Here's how the part is built. I have some questions about the finished solid (model axes, mm). Coordinates: 2 decimals unless noted, no trailing zeros. Write each loop counter-clockwise with the first axis right and the second up, starting at its lowest first coordinate (ties: lowest second). Pieces come first, ordered by that corner, then holes. Notation, with made-up numbers: (-24, 89.5) -> (10, 89.5) arc R21 cw to (10, 120.5) -> close; hole circle Ø7 at (62.5, -21). An arc over 180 degrees is marked (long way). Use a Markdown table: item, result. Add a question column.
Item 1: Imagine slicing it at A-A, the plane x = 5.75. Write out the boundary of the cut face in (y, z).
Item 2: Will this pin go through, and if not, where does the flat tip stop? pin 1 Ø9 at (x, y) = (11.5, -1519.5) entering from +Z.
Item 3: Imagine slicing it at B-B, the plane y = -153. Write out the boundary of the cut face in (x, z).
Item 4: If I drill on line 1 along Y through (x, z) = (9, 227); line 2 along Z through (x, y) = (15.5, -1504), over which ranges is the centre line in solid material (lowest first)? Write a range as from..to.
```python
from build123d import *

# Parameters (mm, degrees)
F0_W     = 17.78
F0_H     = 241.3
F1_DEPTH = 1778
F2_W     = 177.8
F2_H     = 25.4
F3_DEPTH = 17.781


with BuildPart() as f1:
    # F0 (on Front) → F1 (new body)
    with BuildSketch(Plane.XZ):
        with Locations((8.89, 120.65)):
            Rectangle(F0_W, F0_H)
    extrude(amount=F1_DEPTH)

    # F2 (on face) → F3 (cut, through all)
    with BuildSketch(Plane.YZ.offset(17.78)):
        with Locations((-203.2, 228.6)):
            Rectangle(F2_W, F2_H)
        with Locations((-1555.75, 228.6)):
            Rectangle(F2_W, F2_H)
    extrude(amount=-F3_DEPTH, mode=Mode.SUBTRACT)


solid = f1.part
```
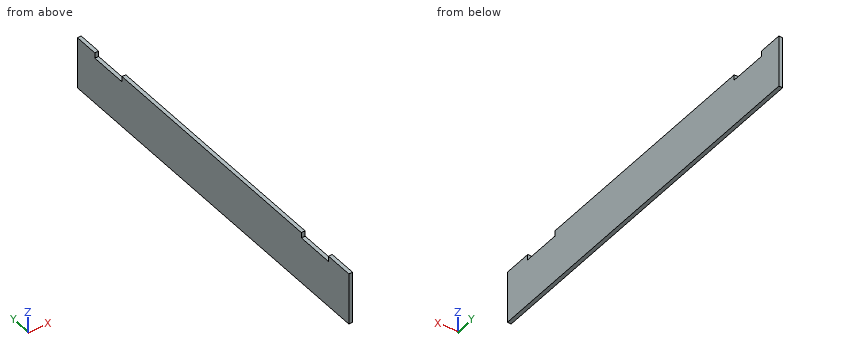
Ans:
| question | item | result |
|---|---|---|
| 1 | outline | (-1778, 0) -> (0, 0) -> (0, 241.3) -> (-114.3, 241.3) -> (-114.3, 215.9) -> (-292.1, 215.9) -> (-292.1, 241.3) -> (-1466.85, 241.3) -> (-1466.85, 215.9) -> (-1644.65, 215.9) -> (-1644.65, 241.3) -> (-1778, 241.3) -> close |
| 2 | pin 1 | stops at z = 215.9 |
| 3 | outline | (0, 0) -> (17.78, 0) -> (17.78, 215.9) -> (0, 215.9) -> close |
| 4 | line 1 | y = -1778..-1644.65, -1466.85..-292.1, -114.3..0 |
| 4 | line 2 | z = 0..215.9 |
